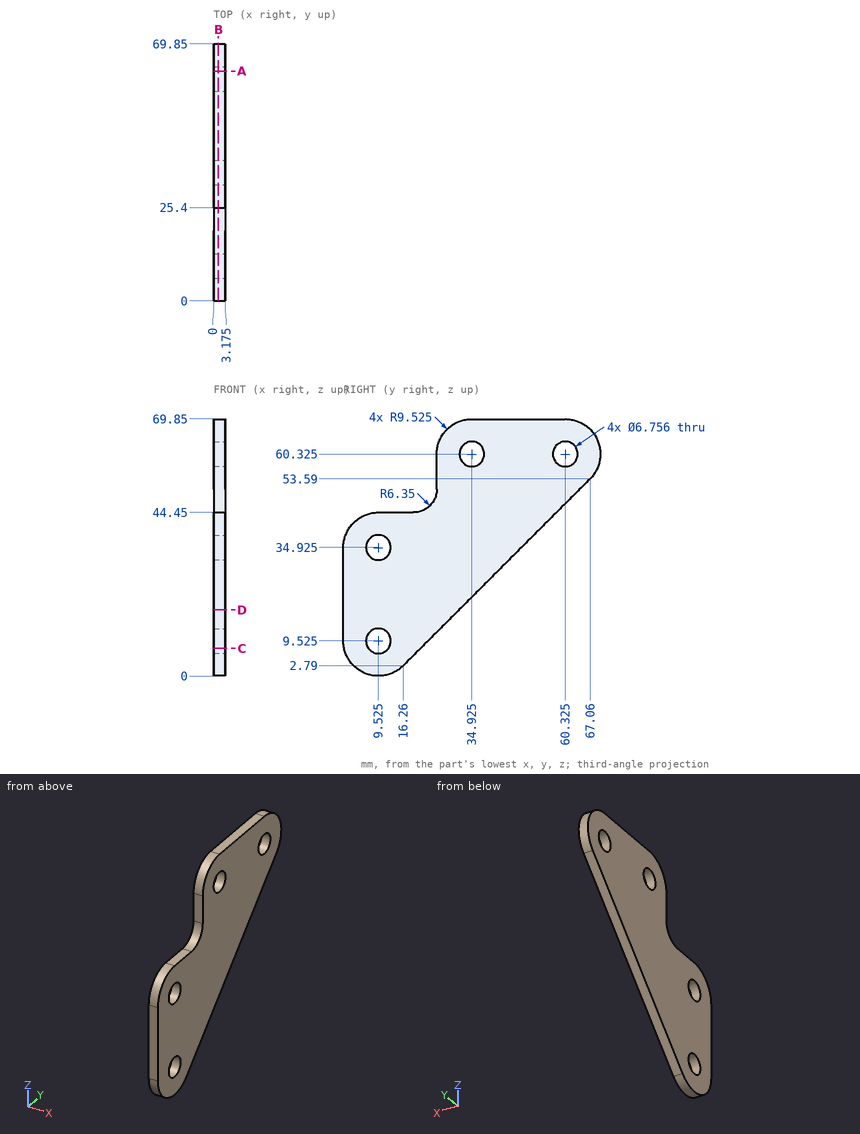
Verification items for this drawing (mm, ordinates from the low corner). Coordinates: 2 decimals unless noted, no trailing zeros. Loops run counter-clockwise (first coordinate to the right, second up) from the corner with the lowest first, then second, coordinate; pieces in that order, holes last. Notation, with made-up numbers: (9.5, 74.5) -> (27.5, 74.5) arc R26 cw to (27.5, 93.5) -> close; hole circle Ø4 at (60.5, -4). An arc over 180 degrees is marked (long way). Put each result on its own line as item: value.
1. Thickness scan on line 1 (Z direction, x = 0.35, y = 8); line 2 (Z direction, x = 1.4, y = 10); line 3 (Z direction, x = 2.2, y = 58.5). Record the ranges inside material, lowest first.
Result set:
line 1: z = 0.12 to 6.51, 12.54 to 31.91, 37.94 to 44.33
line 2: z = 0.01 to 6.18, 12.87 to 31.58, 38.27 to 44.45
line 3: z = 45.03 to 57.48, 63.17 to 69.85
2. Section check B-B, the plane x = 1.25. Give the number of separate pieces and of enclosed holes in the cut face, then the cut area to 3 significant figures.
Result set:
separate pieces: 1
enclosed holes: 4
area: 2,430 mm^2
3. Gauge pin test, flat ends, axial feed: P1, Ø1, axis at x = 2, y = 12, coming from the +Z side; P2, Ø1.5, axis at x = 2, y = 53.5, coming from the -Z side; P3, Ø6, axis at y = 60.325, z = 60.325, coming from the -X side; P4, Ø1.5, axis at x = 0.5, z = 14.5, coming from the +Y side. Record the tip position at first contact, or that the pin passes through.
Result set:
P1: stops at z = 44.45
P2: stops at z = 39.28
P3: passes through
P4: stops at y = 28.72
4. Section check A-A, the plane y = 62.5. Record the boundary of the cut face in (x, z) (1 decimal).
Result set:
outline: (0, 49) -> (3.2, 49) -> (3.2, 57.7) -> (0, 57.7) -> close; (0, 62.9) -> (3.2, 62.9) -> (3.2, 69.6) -> (0, 69.6) -> close
5. Section check C-C, the plane z = 7.5. Record the boundary of the cut face in (x, y) (1 decimal).
Result set:
outline: (0, 0.2) -> (3.2, 0.2) -> (3.2, 6.8) -> (0, 6.8) -> close; (0, 12.2) -> (3.2, 12.2) -> (3.2, 21) -> (0, 21) -> close
6. Section check D-D, the plane z = 18. Record the boundary of the cut face in (x, y) (1 decimal).
Result set:
outline: (0, 0) -> (3.2, 0) -> (3.2, 31.5) -> (0, 31.5) -> close
